Verification items for this drawing (mm, ordinates from the low corner). Give positions to 0.01 mm unless a question says otherwise; leave off trailing zeros. Order: outer loops, then holes, each group sorted by start corner. A loop starts at its lowest first (then second) coordinate and runs counter-clockwise, first axis right, second up.
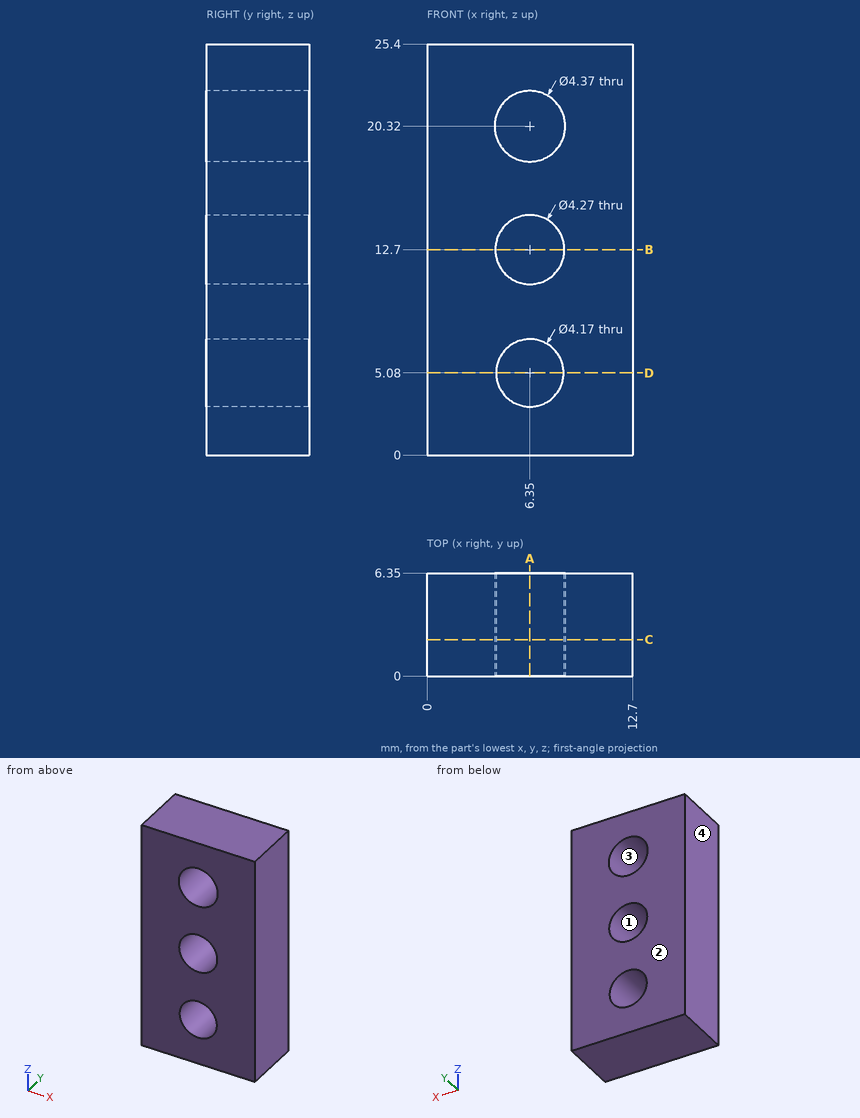
Q1. Cross-section at A-A, the plane x = 6.35. Record the boundary of the cut face in (y, z) (3 decimals), and give its area (3 significant figures).
Q2. Thickness scan on L1, parallel to Z at x = 6.35, y = 2.25 (3 decimals); L2, parallel to Z at x = 7.25, y = 4.25; L3, parallel to X at y = 4, z = 12.7 (3 decimals). Record the ranges inside material, lowest first.
Q3. Cross-section at D-D, the plane z = 5.08. Record the boundary of the cut face in (x, y) (3 decimals), and give its area (3 significant figures).
Q4. Release check for a two-part mould opening along X. For the marked faces 1, 2, 3 and 4 record: pulls with the +X half, pulls with the -X half, needs draft (parallel to the pull), parting line crosses it, or undercut.
Q5. Cross-section at C-C, the plane y = 2.25. Record the boundary of the cut face in (x, z) (3 decimals), and give its area (3 significant figures).
Q6. Cross-section at B-B, the plane z = 12.7. Record the boundary of the cut face in (x, y) (3 decimals).
Answers follow:
1. outline: (0, 0) - (6.35, 0) - (6.35, 2.995) - (0, 2.995) - close; (0, 7.165) - (6.35, 7.165) - (6.35, 10.565) - (0, 10.565) - close; (0, 14.835) - (6.35, 14.835) - (6.35, 18.135) - (0, 18.135) - close; (0, 22.505) - (6.35, 22.505) - (6.35, 25.4) - (0, 25.4) - close
1. area: 79.9 mm2
2. L1: z = 0 to 2.995, 7.165 to 10.565, 14.835 to 18.135, 22.505 to 25.4
2. L2: z = 0 to 3.2, 6.96 to 10.76, 14.64 to 18.33, 22.31 to 25.4
2. L3: x = 0 to 4.215, 8.485 to 12.7
3. outline: (0, 0) - (4.265, 0) - (4.265, 6.35) - (0, 6.35) - close; (8.435, 0) - (12.7, 0) - (12.7, 6.35) - (8.435, 6.35) - close
3. area: 54.2 mm2
4. face 1: undercut
4. face 2: needs draft
4. face 3: undercut
4. face 4: pulls with the -X half
5. outline: (0, 0) - (12.7, 0) - (12.7, 25.4) - (0, 25.4) - close; hole circle Ø4.37 at (6.35, 20.32); hole circle Ø4.27 at (6.35, 12.7); hole circle Ø4.17 at (6.35, 5.08)
5. area: 280 mm2
6. outline: (0, 0) - (4.215, 0) - (4.215, 6.35) - (0, 6.35) - close; (8.485, 0) - (12.7, 0) - (12.7, 6.35) - (8.485, 6.35) - close
